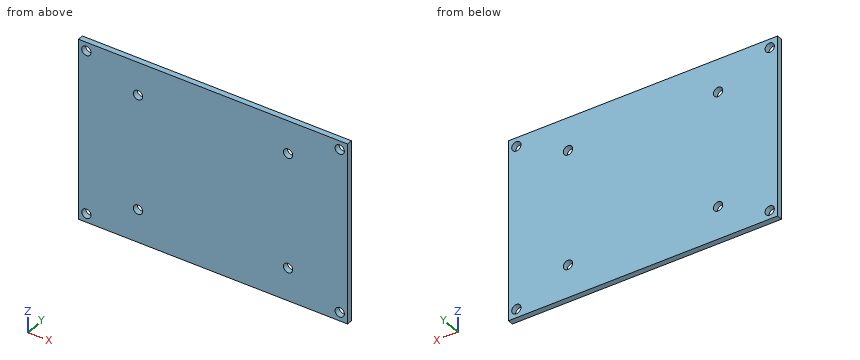
```python
from build123d import *

# Parameters (mm, degrees)
CROQUIS7_W                   = 75.3
CROQUIS7_H                   = 50.3
SALIENTE_EXTRUIR1_DEPTH      = 1.6
TALADRO_DE_MARGEN_PARA_M23_D = 2.6
TALADRO_DE_MARGEN_PARA_M24_D = 2.6


with BuildPart() as part:
    # Croquis7 → Saliente-Extruir1 (new body)
    with BuildSketch(Plane(origin=(0, 0, 0), x_dir=(1, 0, 0), z_dir=(0, 1, 0))):
        Rectangle(CROQUIS7_W, CROQUIS7_H)
    extrude(amount=SALIENTE_EXTRUIR1_DEPTH)

    # Taladro de margen para M23 (through all)
    with Locations(Plane(origin=(0, 1.6, 0), x_dir=(1, 0, 0), z_dir=(0, 1, 0))):
        with Locations((-35.45, 22.75), (35.45, 22.75), (35.45, -22.75), (-35.45, -22.75)):
            Hole(TALADRO_DE_MARGEN_PARA_M23_D / 2)

    # Taladro de margen para M24 (through all)
    with Locations(Plane(origin=(0, 1.6, 0), x_dir=(1, 0, 0), z_dir=(0, 1, 0))):
        with Locations((-21, 16), (21, 16), (21, -16), (-21, -16)):
            Hole(TALADRO_DE_MARGEN_PARA_M24_D / 2)


solid = part.part
```
Build history of the part. All positions in model axes, mm. Round coordinates to 2 decimals unless told otherwise and drop trailing zeros. Write each loop counter-clockwise with the first axis right and the second up, starting at its lowest first coordinate (ties: lowest second). Pieces come first, ordered by that corner, then holes. Notation, with made-up numbers: (1.5, 47.25) - (59.5, 47.25) arc R21 cw to (59.5, 73.25) - close; hole circle Ø10 at (53, -13.5). An arc over 180 degrees is marked (long way). Answer as CSV lines item,"result".
Q1. Drill centre lines: probe 1 along Z at (x, y) = (35.45, 0.4); probe 2 along X at (y, z) = (0.9, -16); probe 3 along X at (y, z) = (0.5, 22.75). Where is each one in solid material? Low to high. Write a range as [from, to].
Report:
probe 1,"z = [-25.15, -24.05], [-21.45, 21.45], [24.05, 25.15]"
probe 2,"x = [-37.65, -22.3], [-19.7, 19.7], [22.3, 37.65]"
probe 3,"x = [-37.65, -36.75], [-34.15, 34.15], [36.75, 37.65]"
Q2. Cut at B-B (x = 35.45). Write the cut outline in (y, z), and give its area (3 significant figures).
Report:
outline,"(0, -25.15) - (1.6, -25.15) - (1.6, -24.05) - (0, -24.05) - close; (0, -21.45) - (1.6, -21.45) - (1.6, 21.45) - (0, 21.45) - close; (0, 24.05) - (1.6, 24.05) - (1.6, 25.15) - (0, 25.15) - close"
area,"72.2 mm^2"
Q3. Drop a flat-ended pin along its axis: pin 1 (3 mm diameter, centred on x = 21, z = -16, fed in from +Y). Give the stop position or say it passes through.
Report:
pin 1,"stops at y = 1.6"
Q4. Cut at A-A (z = -22.75). Write the cut outline in (x, y).
Report:
outline,"(-37.65, 0) - (-36.75, 0) - (-36.75, 1.6) - (-37.65, 1.6) - close; (-34.15, 0) - (34.15, 0) - (34.15, 1.6) - (-34.15, 1.6) - close; (36.75, 0) - (37.65, 0) - (37.65, 1.6) - (36.75, 1.6) - close"
